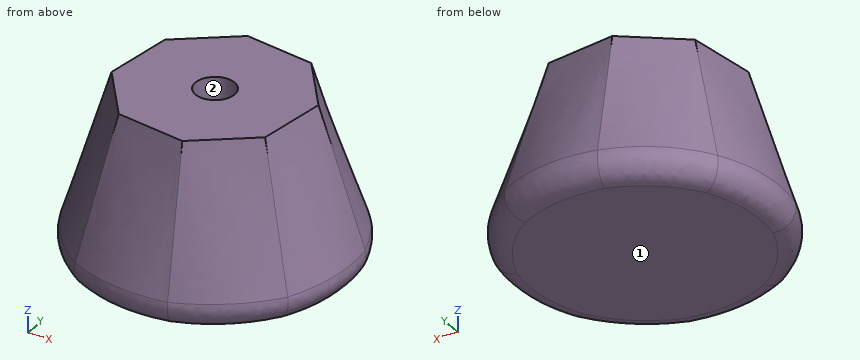
```python
from build123d import *

# Parameters (mm, degrees)
F4_D     = 2.4
F4_DEPTH = 5
F4_TIP   = 0.7210327428
F5_R     = 1.27


# Not quite as in the source:
# - the arcs of a loft's sections are written as splines that run evenly, so that the points pair up as in the source's solid


with BuildPart() as f3:
    # F0 (on Top) → F3 section 0
    with BuildSketch(Plane.XY):
        with BuildLine():
            add(Edge.make_bspline(
                [(2.1287545667, -8.4725466174), (3.2378083255, -8.1938932963), (4.2910199355, -7.694831903), (6.1270120531, -6.3311147047), (6.9090701762, -5.4669954641), (7.4962519567, -4.4857383775)],
                knots=[0, 0, 0, 0, 0.5, 0.5, 1, 1, 1, 1], degree=3))
            add(Edge.make_bspline(
                [(7.4962519567, -4.4857383775), (8.0834337372, -3.504481291), (8.4752771134, -2.4068585241), (8.8092259113, -0.144322369), (8.7511999386, 1.0197008079), (8.4725466174, 2.1287545667)],
                knots=[0, 0, 0, 0, 0.5, 0.5, 1, 1, 1, 1], degree=3))
            add(Edge.make_bspline(
                [(8.4725466174, 2.1287545667), (8.1938932963, 3.2378083255), (7.694831903, 4.2910199355), (6.3311147047, 6.1270120531), (5.4669954641, 6.9090701762), (4.4857383775, 7.4962519567)],
                knots=[0, 0, 0, 0, 0.5, 0.5, 1, 1, 1, 1], degree=3))
            add(Edge.make_bspline(
                [(4.4857383775, 7.4962519567), (3.504481291, 8.0834337372), (2.4068585241, 8.4752771134), (0.144322369, 8.8092259113), (-1.0197008079, 8.7511999386), (-2.1287545667, 8.4725466174)],
                knots=[0, 0, 0, 0, 0.5, 0.5, 1, 1, 1, 1], degree=3))
            add(Edge.make_bspline(
                [(-2.1287545667, 8.4725466174), (-3.2378083255, 8.1938932963), (-4.2910199355, 7.694831903), (-6.1270120531, 6.3311147047), (-6.9090701762, 5.4669954641), (-7.4962519567, 4.4857383775)],
                knots=[0, 0, 0, 0, 0.5, 0.5, 1, 1, 1, 1], degree=3))
            add(Edge.make_bspline(
                [(-7.4962519567, 4.4857383775), (-8.0834337372, 3.504481291), (-8.4752771134, 2.4068585241), (-8.8092259113, 0.144322369), (-8.7511999386, -1.0197008079), (-8.4725466174, -2.1287545667)],
                knots=[0, 0, 0, 0, 0.5, 0.5, 1, 1, 1, 1], degree=3))
            add(Edge.make_bspline(
                [(-8.4725466174, -2.1287545667), (-8.1938932963, -3.2378083255), (-7.694831903, -4.2910199355), (-6.3311147047, -6.1270120531), (-5.4669954641, -6.9090701762), (-4.4857383775, -7.4962519567)],
                knots=[0, 0, 0, 0, 0.5, 0.5, 1, 1, 1, 1], degree=3))
            add(Edge.make_bspline(
                [(-4.4857383775, -7.4962519567), (-3.504481291, -8.0834337372), (-2.4068585241, -8.4752771134), (-0.144322369, -8.8092259113), (1.0197008079, -8.7511999386), (2.1287545667, -8.4725466174)],
                knots=[0, 0, 0, 0, 0.5, 0.5, 1, 1, 1, 1], degree=3))
        make_face()
    # F2 (on offset) → F3 section 1
    with BuildSketch(Plane.XY.offset(10)):
        Polygon((1.3828789294, -5.5039253369), (4.8697059974, -2.9140198603), (5.5039253369, 1.3828789294), (2.9140198603, 4.8697059974), (-1.3828789294, 5.5039253369), (-4.8697059974, 2.9140198603), (-5.5039253369, -1.3828789294), (-2.9140198603, -4.8697059974), align=None)
    loft(ruled=True)

    # F4
    with Locations(Plane.XY.offset(10)):
        with Locations((0, 0)):
            Hole(F4_D / 2, depth=F4_DEPTH)
            with Locations((0, 0, -(F4_DEPTH + F4_TIP / 2))):  # 118° drill point
                Cone(0, F4_D / 2, F4_TIP, mode=Mode.SUBTRACT)

    # F5
    f5_edges = [f3.edges().sort_by_distance(p)[0] for p in [
        (5.209016, -7.012973, 0),
        (8.642252, -1.27559, 0),
        (7.012973, 5.209016, 0),
        (1.27559, 8.642252, 0),
        (-5.209016, 7.012973, 0),
        (-8.642252, 1.27559, 0),
        (-7.012973, -5.209016, 0),
        (-1.27559, -8.642252, 0),
    ]]
    fillet(f5_edges, radius=F5_R)


solid = f3.part
```
Work out the finished part from the listing and answer in its coordinate system (mm). Face numbers are marked on the shaded views. Round coordinates to 2 decimals unless told otherwise and drop trailing zeros.
1) Flat-ended cylindrical pins translate along their axes: P1, Ø1.5, axis at x = 4, z = 3.5, coming from the +Y side; P2, Ø6, axis at x = -1, z = 4, coming from the -Y side; P3, Ø1, axis at y = 4.5, z = 4.5, coming from the +X side; P4, Ø1, axis at y = -2.5, z = 1.5, coming from the +X side. Find the tip coordinate at first contact, or state that the pin passes through.
2) Consider probe 1 along Y at (x, z) = (0, 7.45); probe 2 along Y at (x, z) = (0, 6.05); probe 3 along X at (y, z) = (0, 8.9). Determine where each line is inside the solid, lowest interval first.
3) Determine the mould class of the marked faces 1 and 2 for opening direction X: pulls with the +X half, pulls with the -X half, needs draft (parallel to the pull), parting line crosses it, or undercut.
Entries:
1. P1: stops at y = 6.97
1. P2: stops at y = -8.23
1. P3: stops at x = 6.01
1. P4: stops at x = 7.97
2. probe 1: y = -6.18 to -1.2, 1.2 to 6.18
2. probe 2: y = -6.66 to -1.2, 1.2 to 6.66
2. probe 3: x = -5.68 to -1.2, 1.2 to 5.68
3. face 1: needs draft
3. face 2: undercut
